Check sheet for the drawn part. Datum: minimum x, y, z corner. Units: mm. Round coordinates to 2 decimals unless told otherwise and drop trailing zeros. Write each loop counter-clockwise with the first axis right and the second up, starting at its lowest first coordinate (ties: lowest second). Pieces come first, ordered by that corner, then holes. Notation, with made-up numbers: (28.5, 77) - (72.5, 77) arc R18 cw to (72.5, 81) - close; hole circle Ø4 at (-34, 64). An arc over 180 degrees is marked (long way). Answer as a JSON object with one key per item and string values. Group by question number.
1) Mould release check, pull along X, two halves, no side actions. Record for the marked faces 1, 2 and 3: +X half, -X half, draft (parallel to the pull), parting line (faces both ways), or undercut.
2) Section check B-B (y = 4). Enter the section's corners in (x, z), then the cut area to 3 significant figures.
3) Section check C-C (z = 12.75). Enter the section's corners in (x, y), then the cut area to 3 significant figures.
4) Thickness scan on line 1 (Y direction, x = 25, z = 13.15); line 2 (X direction, y = 25.5, z = 12.75) (3 decimals); line 3 (Z direction, x = 23.5, y = 13). Record the ranges inside material, lowest first.
5) Go/stop test with flat-tipped pins: pin 1 Ø6 at (y, z) = (30, 7.5) entering from -X; pin 2 Ø1.8 at (x, y) = (47, 25) entering from +Z; pin 3 Ø1 at (x, z) = (22, 2) entering from -Y; pin 4 Ø1 at (y, z) = (26, 12.5) entering from +X (3 decimals). Record where each tip stops, or that it passes through.
6) Section check A-A (x = 5). Enter the section's corners in (y, z), then the cut area to 3 significant figures.
7) Section check D-D (x = 40). Enter the section's corners in (y, z), then the cut area to 3 significant figures.
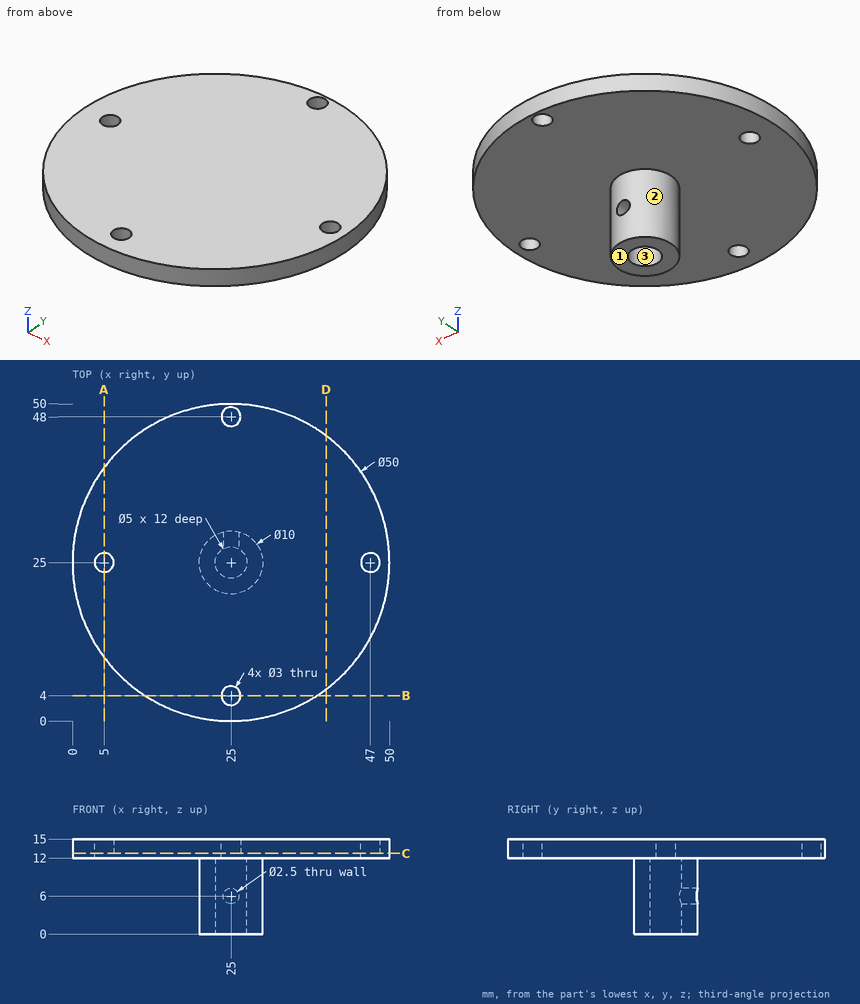
Returned:
{
 "1": {"face 1": "draft", "face 2": "parting line", "face 3": "undercut"},
 "2": {"outline": "(11.44, 12) - (23.5, 12) - (23.5, 15) - (11.44, 15) - close; (26.5, 12) - (38.56, 12) - (38.56, 15) - (26.5, 15) - close", "area": "72.4 mm2"},
 "3": {"outline": "circle Ø50 at (25, 25); hole circle Ø3 at (5, 25); hole circle Ø3 at (25, 4); hole circle Ø3 at (25, 48); hole circle Ø3 at (47, 25)", "area": "1,940 mm2"},
 "4": {"line 1": "0 to 2.5, 5.5 to 46.5, 49.5 to 50", "line 2": "0.005 to 3.586, 6.414 to 45.586, 48.414 to 49.995", "line 3": "12 to 15"},
 "5": {"pin 1": "x = 20.42", "pin 2": "through", "pin 3": "y = 20.67", "pin 4": "x = 49.995"},
 "6": {"outline": "(10, 12) - (23.5, 12) - (23.5, 15) - (10, 15) - close; (26.5, 12) - (40, 12) - (40, 15) - (26.5, 15) - close", "area": "81.0 mm2"},
 "7": {"outline": "(5, 12) - (45, 12) - (45, 15) - (5, 15) - close", "area": "120 mm2"}
}
